Here's how the part is built. I have some questions about the finished solid (model axes, mm). A direction names the side the tool comes from. Give positions to 0.01 mm unless a question says otherwise; leave off trailing zeros. Loops run counter-clockwise (first coordinate to the right, second up) from the corner with the lowest first, then second, coordinate; pieces in that order, holes last.
Q1. Thinking about a two-plate mould opening in X: for faces 3 (the face through (96, 2, 30)), 4 (the face through (151.185, 1.521, 16.201)), 5 (the face through (195, 8.3, 2.8)), which applies, pulls with the +X half, pulls with the -X half, needs draft (parallel to the pull), parting line crosses it, or undercut?
Q2. I need wall thicknesses on probe 1 along X at (y, z) = (20, 2.4); probe 2 along Z at (x, y) = (155, 1.4); probe 3 along Y at (x, z) = (15, 2.3). Which ranges of each line are inside material? Lowest first, please.
Q3. Suppose I cut it at A-A (x = 15). List the corners of the cut face in (y, z) for me, and give its area (3 significant figures).
Q4. For faces 1 (the face through (96, 3, 16)), 2 (the face through (96, 30, 1)), which set-ups out of +Z, -Z, +X, -X, +Y, -Y let a thin tool reach every point of the face, with its end or its side?
Q5. I'm going to push flat-ended pins straight in: P1, Ø13.5, axis at x = 99, z = 15, coming from the +Y side; P2, Ø12, axis at y = 17.5, z = 11.5, coming from the -X side; P3, Ø12, axis at x = 144, y = 20, coming from the -Z side; P4, Ø10, axis at x = 149, y = 21.5, coming from the +Z side. Where does each tip first touch, or does it pass through?
Q6. Suppose I cut it at C-C (x = 161). List the corners of the cut face in (y, z) for me.
Q7. Suppose I cut it at B-B (y = 17.75). List the corners of the cut face in (x, z) for me.
```python
from build123d import *

# Parameters (mm, degrees)
F1_DEPTH = 195
F3_D     = 8
F5_D     = 8


with BuildPart() as f1:
    # F0 (on Right) → F1 (new body)
    with BuildSketch(Plane.YZ):
        Polygon((0, 30), (0, 0), (30, 0), (30, 3), (3, 3), (3, 30), align=None)
    extrude(amount=F1_DEPTH)

    # F3 (through all)
    with Locations(Plane(origin=(0, 0, 0), x_dir=(1, 0, 0), z_dir=(0, 0, -1))):
        with Locations((15, -20), (170, -20)):
            Hole(F3_D / 2)

    # F5 (through all)
    with Locations(Plane.XZ):
        with Locations((30, 15), (155, 15)):
            Hole(F5_D / 2)


solid = f1.part
```
Solutions:
1. face 3: needs draft
1. face 4: undercut
1. face 5: pulls with the +X half
2. probe 1: x = 0 to 11, 19 to 166, 174 to 195
2. probe 2: z = 0 to 11, 19 to 30
2. probe 3: y = 0 to 16, 24 to 30
3. outline: (0, 0) - (16, 0) - (16, 3) - (3, 3) - (3, 30) - (0, 30) - close; (24, 0) - (30, 0) - (30, 3) - (24, 3) - close
3. area: 147 mm2
4. face 1: +Z, +X, -X, +Y
4. face 2: +Z, -Z, +X, -X, +Y
5. P1: stops at y = 3
5. P2: passes through
5. P3: stops at z = 0
5. P4: stops at z = 3
6. outline: (0, 0) - (30, 0) - (30, 3) - (3, 3) - (3, 30) - (0, 30) - close
7. outline: (0, 0) - (11.69, 0) - (11.69, 3) - (0, 3) - close; (18.31, 0) - (166.69, 0) - (166.69, 3) - (18.31, 3) - close; (173.31, 0) - (195, 0) - (195, 3) - (173.31, 3) - close
